```python
from build123d import *

# Parameters (mm, degrees)
EXTRUDE_1_DEPTH               = 175
EXTRUDE_1_DEPTH_BACK          = 175
SKETCH_2_W                    = 30
SKETCH_2_H                    = 24
CUT_EXTRUDE_1_DEPTH           = 212.186188109
SKETCH_3_R                    = 8
SKETCH_3_R_2                  = 10
CUT_EXTRUDE_2_DEPTH           = 200.099487814
SKETCH_4_W                    = 162
SKETCH_4_H                    = 18
CUT_EXTRUDE_3_DEPTH           = 212.186188109
SKETCH_9_R                    = 8
CUT_EXTRUDE_8_DEPTH           = 197.23996604
CHAMFER_1_SIZE                = 20
CHAMFER_2_SIZE                = 5
HOLE_WIZARD_M16_1_D           = 17
HOLE_WIZARD_M16_1_CBORE_D     = 26
HOLE_WIZARD_M16_1_CBORE_DEPTH = 20
PATTERN_LINEAR_1_COUNT        = 3
PATTERN_LINEAR_1_PITCH        = 140
PATTERN_LINEAR_1_COUNT_DIR2   = 2
PATTERN_LINEAR_1_PITCH_DIR2   = 30
M6X1_0_1_D                    = 5
M6X1_0_1_DEPTH                = 15
M6X1_0_1_TIP                  = 1.502151548


with BuildPart() as part:
    # 草图1 → 拉伸1 (new, two sides: drawn at the far end of the back side and taken through both)
    with BuildSketch(Plane.XY.offset(-EXTRUDE_1_DEPTH_BACK)):
        Polygon((-46.669668375, 36.955523256), (53.330331625, 36.955523256), (53.330331625, 7.955523256), (-17.669668375, 7.955523256), (-17.669668375, -63.044476744), (-46.669668375, -63.044476744), align=None)
    extrude(amount=EXTRUDE_1_DEPTH + EXTRUDE_1_DEPTH_BACK)

    # 草图2 → 切除-拉伸1 (cut, through all)
    with BuildSketch(Plane.ZY.offset(46.669668375)):
        with Locations((160, -29.044476744)):
            Rectangle(SKETCH_2_W, SKETCH_2_H)
    cut_extrude_1 = extrude(amount=-CUT_EXTRUDE_1_DEPTH, mode=Mode.SUBTRACT)

    # 镜向1: 切除-拉伸1 across plane
    add(cut_extrude_1.mirror(Plane.XY), mode=Mode.SUBTRACT)

    # 草图3 → 切除-拉伸2 (cut, through all)
    with BuildSketch(Plane(origin=(-17.669668375, 0, 0), x_dir=(0, 0, -1), z_dir=(1, 0, 0))):
        with Locations(Location((0, -29.044476744, 0), (0, 0, 90))):
            Circle(SKETCH_3_R)
        with Locations(Location((100, -29.044476744, 0), (0, 0, 90))):
            Circle(SKETCH_3_R_2)
        with Locations(Location((-100, -29.044476744, 0), (0, 0, 90))):
            Circle(SKETCH_3_R_2)
    extrude(amount=-CUT_EXTRUDE_2_DEPTH, mode=Mode.SUBTRACT)

    # 草图4 → 切除-拉伸3 (cut, through all)
    with BuildSketch(Plane.ZY.offset(46.669668375)):
        with Locations((0, -54.044476744)):
            Rectangle(SKETCH_4_W, SKETCH_4_H)
    extrude(amount=-CUT_EXTRUDE_3_DEPTH, mode=Mode.SUBTRACT)

    # 草图9 → 切除-拉伸8 (cut, through all)
    with BuildSketch(Plane.XZ.offset(-7.955523256)):
        with Locations(Location((17.330331625, -90, 0), (0, 0, 270))):
            Circle(SKETCH_9_R)
        with Locations(Location((17.330331625, 90, 0), (0, 0, 270))):
            Circle(SKETCH_9_R)
    extrude(amount=-CUT_EXTRUDE_8_DEPTH, mode=Mode.SUBTRACT)

    # 倒角1
    chamfer_1_edges = [part.edges().sort_by_distance(p)[0] for p in [
        (53.330331625, 22.455523256, -175),
        (53.330331625, 22.455523256, 175),
    ]]
    chamfer(chamfer_1_edges, length=CHAMFER_1_SIZE)

    # 倒角2
    chamfer_2_edges = [part.edges().sort_by_distance(p)[0] for p in [
        (-32.169668375, -63.044476744, 175),
        (-32.169668375, -63.044476744, -175),
        (-32.169668375, -17.044476744, 175),
        (-32.169668375, -41.044476744, 175),
        (-32.169668375, -41.044476744, -175),
        (-32.169668375, -17.044476744, -175),
        (-32.169668375, -63.044476744, -81),
        (-32.169668375, -63.044476744, 81),
    ]]
    chamfer(chamfer_2_edges, length=CHAMFER_2_SIZE)

    # M16 六角凹头螺钉的柱形沉头孔1 (through all)
    with Locations(Plane.XZ.offset(-7.955523256)):
        with Locations((2.330331625, -140)):
            hole_wizard_m16_1 = CounterBoreHole(HOLE_WIZARD_M16_1_D / 2, HOLE_WIZARD_M16_1_CBORE_D / 2, HOLE_WIZARD_M16_1_CBORE_DEPTH)

    # 阵列(线性)1: Hole Wizard M16 _1 3 × 2
    with Locations(*[(j * PATTERN_LINEAR_1_PITCH_DIR2, 0, i * PATTERN_LINEAR_1_PITCH) for i in range(PATTERN_LINEAR_1_COUNT) for j in range(PATTERN_LINEAR_1_COUNT_DIR2) if (i, j) != (0, 0)]):
        add(hole_wizard_m16_1, mode=Mode.SUBTRACT)

    # M6x1.0 螺纹孔1
    with Locations(Plane.ZY.offset(46.669668375)):
        with Locations((80, 0), (-80, 0)):
            Hole(M6X1_0_1_D / 2, depth=M6X1_0_1_DEPTH)
            with Locations((0, 0, -(M6X1_0_1_DEPTH + M6X1_0_1_TIP / 2))):  # 118° drill point
                Cone(0, M6X1_0_1_D / 2, M6X1_0_1_TIP, mode=Mode.SUBTRACT)


solid = part.part
```
Geometry: final body of the model. Coordinates: model frame, mm. A direction names the side the tool comes from. Coordinates: 2 decimals unless noted, no trailing zeros. Loops run counter-clockwise (first coordinate to the right, second up) from the corner with the lowest first, then second, coordinate; pieces in that order, holes last. Notation, with made-up numbers: (24, -27.75) -> (28, -27.75) arc R11 ccw to (28, -6.75) -> close; hole circle Ø3 at (51.25, 33). An arc over 180 degrees is marked (long way). Use a Markdown table: item, result. Add a question column.
(1) Section query A-A, the plane y = -51. Return loops of the section in (x, z).
(2) Pin query (flat end, axial travel): pin 1 Ø21 at (x, z) = (38.5, 137) entering from -Y; pin 2 Ø6.5 at (y, z) = (0, -80) entering from +X; pin 3 Ø19 at (x, y) = (-35.5, -24.5) entering from -Z; pin 4 Ø4 at (x, y) = (-10, 7.5) entering from +Z. Return the tip coordinate at first contact, or that it passes through.
(3) Section query D-D, the plane y = -34. Return loops of the section in (x, z).
(4) Access query for faces 1 (the cylindrical face through (-0.49, 17.82, -12.69)), 2 (the flat face through (-32, -52, 81)), 3 (the flat face through (-32, -41.044, 157)). Directions: +Z, -Z, +X, -X, +Y, -Y. A direction counts if a zero-diameter tool reaches every point of the face in a straight line with its end or side. Return the directions, or none.
(5) Line query: line 1 along Z through (x, y) = (-7.5, 10); line 2 along Z through (x, y) = (-34.5, -28.5); line 3 along Z through (x, y) = (-39.5, -53). Output: solid intervals per line, ascending.
(6) Mould query, pull axis X, two halves, no side actions, for faces 4 (the cylindrical face through (-31.967, -30.346, 109.915)), 5 (the flat face through (-17.67, -19, -2)), 6 (the cylindrical face through (12.462, 22.253, 96.349)), 7 (the cylindrical face through (-0.49, 17.82, -152.69)). Classes: pulls with the +X half, pulls with the -X half, needs draft (parallel to the pull), parting line crosses it, or undercut.
(7) Section query B-B, the plane z = 0. Return loops of the section in (x, y), plus the area to 3 significant figures.
(8) Section query C-C, the plane x = -26. Return loops of the section in (y, z), plus the area to 3 significant figures.
Answer:
| question | item | result |
|---|---|---|
| 1 | outline | (-46.67, -175) -> (-17.67, -175) -> (-17.67, -81) -> (-46.67, -81) -> close; (-46.67, 81) -> (-17.67, 81) -> (-17.67, 175) -> (-46.67, 175) -> close |
| 2 | pin 1 | stops at y = 7.96 |
| 2 | pin 2 | stops at x = -17.67 |
| 2 | pin 3 | stops at z = -172.04 |
| 2 | pin 4 | stops at z = 175 |
| 3 | outline | (-46.67, -145) -> (-17.67, -145) -> (-17.67, -108.69) -> (-46.67, -108.69) -> close; (-46.67, -91.31) -> (-17.67, -91.31) -> (-17.67, -6.28) -> (-46.67, -6.28) -> close; (-46.67, 6.28) -> (-17.67, 6.28) -> (-17.67, 91.31) -> (-46.67, 91.31) -> close; (-46.67, 108.69) -> (-17.67, 108.69) -> (-17.67, 145) -> (-46.67, 145) -> close |
| 4 | face 1 | -Y |
| 4 | face 2 | +X, -X, -Y |
| 4 | face 3 | +Z, +X, -X |
| 5 | line 1 | z = -175 to -148.51, -131.49 to -8.51, 8.51 to 131.49, 148.51 to 175 |
| 5 | line 2 | z = -145 to -109.99, -90.01 to -7.98, 7.98 to 90.01, 109.99 to 145 |
| 5 | line 3 | z = -175 to -81, 81 to 175 |
| 6 | face 4 | needs draft |
| 6 | face 5 | pulls with the +X half |
| 6 | face 6 | undercut |
| 6 | face 7 | undercut |
| 7 | outline | (-46.67, -45.04) -> (-17.67, -45.04) -> (-17.67, -37.04) -> (-46.67, -37.04) -> close; (-46.67, -21.04) -> (-17.67, -21.04) -> (-17.67, 7.96) -> (-10.67, 7.96) -> (-10.67, 27.96) -> (-6.17, 27.96) -> (-6.17, 36.96) -> (-46.67, 36.96) -> close; (10.83, 27.96) -> (15.33, 27.96) -> (15.33, 7.96) -> (19.33, 7.96) -> (19.33, 27.96) -> (23.83, 27.96) -> (23.83, 36.96) -> (10.83, 36.96) -> close; (40.83, 27.96) -> (45.33, 27.96) -> (45.33, 7.96) -> (53.33, 7.96) -> (53.33, 36.96) -> (40.83, 36.96) -> close |
| 7 | area | 2,630 mm^2 |
| 8 | outline | (-63.04, -170) -> (-58.04, -175) -> (-46.04, -175) -> (-41.04, -170) -> (-41.04, -145) -> (-17.04, -145) -> (-17.04, -170) -> (-12.04, -175) -> (36.96, -175) -> (36.96, 175) -> (-12.04, 175) -> (-17.04, 170) -> (-17.04, 145) -> (-41.04, 145) -> (-41.04, 170) -> (-46.04, 175) -> (-58.04, 175) -> (-63.04, 170) -> (-63.04, 86) -> (-58.04, 81) -> (-45.04, 81) -> (-45.04, -81) -> (-58.04, -81) -> (-63.04, -86) -> close; hole circle Ø20 at (-29.04, -100); hole circle Ø20 at (-29.04, 100); hole circle Ø16 at (-29.04, 0) |
| 8 | area | 29,700 mm^2 |
